Design review of the part built by this model. Coordinates are the model's own, in mm. A direction names the side the tool comes from. Give positions to 0.01 mm unless a question says otherwise; leave off trailing zeros. Loops run counter-clockwise (first coordinate to the right, second up) from the corner with the lowest first, then second, coordinate; pieces in that order, holes last. Notation, with made-up numbers: (-13, 75.5) -> (44, 75.5) arc R21 cw to (44, 114.5) -> close; hole circle Ø1 at (59, 20.25). An arc over 180 degrees is marked (long way). Answer in a Markdown table with one row per item. Add a question column.
(1) Draft analysis for pull direction Y (two halves, no side actions). For faces 1 (the flat face through (216, -6.3, 0)), 2 (the flat face through (216, -7.5, 0)), 3 (the flat face through (216, 0, -8.8)), 4 (the flat face through (216, 0, -10)), state which applies: +Y half, -Y half, draft (parallel to the pull), parting line (faces both ways), or undercut.
(2) Consider section B-B on x = 232.5. Write out the cut boundary in (y, z).
(3) For faces 5 (the flat face through (216, 6.3, 0)), 6 (the flat face through (438, 7, 0)), list the 3-axis set-ups (+Z, -Z, +X, -X, +Y, -Y) from which the entire face can be reached by the end or side of a thin tool; tool diameter is ignored.
(4) For line 1 (X direction, y = -7, z = 0); line 2 (Z direction, x = 348, y = -7.15); line 3 (Y direction, x = 76, z = -7), list the stretches that pass through material, from the lowest coordinate up.
(5) Consider section A-A on y = 4. Write out the cut boundary in (x, z).
from build123d import *

# Parameters (mm, degrees)
SKETCH1_W               = 20
SKETCH1_H               = 15
SKETCH1_W_2             = 17.6
SKETCH1_H_2             = 12.6
F_15_X_20_X_1_2_1_DEPTH = 438
SKETCH_3_R              = 2.5
CUT_EXTRUDE_1_DEPTH     = 439.370847571


with BuildPart() as part:
    # Sketch1 → 方形管 15 X 20 X 1.2(1) (new body)
    with BuildSketch(Plane(origin=(0, 0, 0), x_dir=(0, 0, -1), z_dir=(1, 0, 0))):
        Rectangle(SKETCH1_W, SKETCH1_H)
        Rectangle(SKETCH1_W_2, SKETCH1_H_2, mode=Mode.SUBTRACT)
    extrude(amount=F_15_X_20_X_1_2_1_DEPTH)

    # 草图3 → 切除-拉伸1 (cut, through all)
    with BuildSketch(Plane(origin=(0, 7.5, 0), x_dir=(1, 0, 0), z_dir=(0, 1, 0))):
        with Locations(Location((188, 0, 0), (0, 0, 270))):
            Circle(SKETCH_3_R)
        with Locations(Location((252, 0, 0), (0, 0, 270))):
            Circle(SKETCH_3_R)
        with Locations(Location((348, 0, 0), (0, 0, 270))):
            Circle(SKETCH_3_R)
        with Locations(Location((412, 0, 0), (0, 0, 270))):
            Circle(SKETCH_3_R)
    extrude(amount=-CUT_EXTRUDE_1_DEPTH, mode=Mode.SUBTRACT)


solid = part.part
Values follow:
| question | item | result |
|---|---|---|
| 1 | face 1 | undercut |
| 1 | face 2 | -Y half |
| 1 | face 3 | undercut |
| 1 | face 4 | draft |
| 2 | outline | (-7.5, -10) -> (7.5, -10) -> (7.5, 10) -> (-7.5, 10) -> close; hole (-6.3, -8.8) -> (6.3, -8.8) -> (6.3, 8.8) -> (-6.3, 8.8) -> close |
| 3 | face 5 | +X, -X |
| 3 | face 6 | +Z, -Z, +X, +Y, -Y |
| 4 | line 1 | 0 to 185.5, 190.5 to 249.5, 254.5 to 345.5, 350.5 to 409.5, 414.5 to 438 |
| 4 | line 2 | -10 to -2.5, 2.5 to 10 |
| 4 | line 3 | -7.5 to -6.3, 6.3 to 7.5 |
| 5 | outline | (0, -10) -> (438, -10) -> (438, -8.8) -> (0, -8.8) -> close; (0, 8.8) -> (438, 8.8) -> (438, 10) -> (0, 10) -> close |
